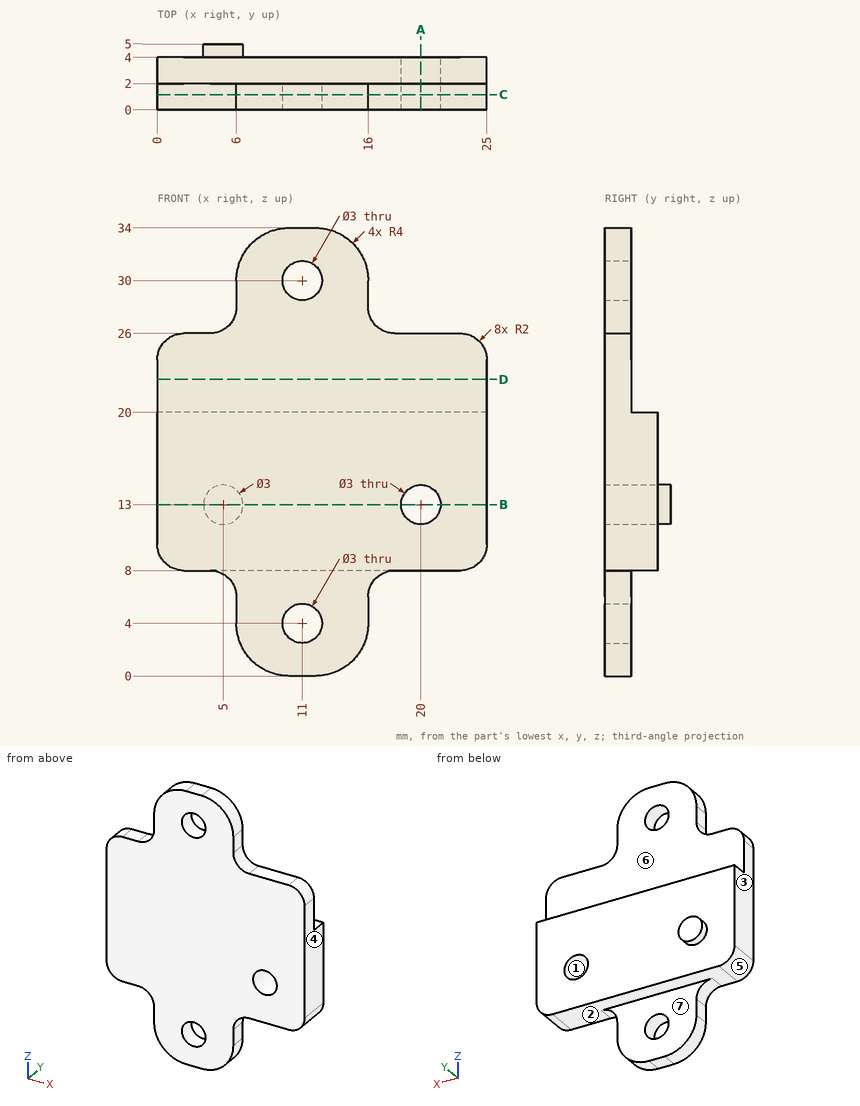
Verification items for this drawing (mm, ordinates from the low corner). A direction names the side the tool comes from. Round coordinates to 2 decimals unless told otherwise and drop trailing zeros. Loops run counter-clockwise (first coordinate to the right, second up) from the corner with the lowest first, then second, coordinate; pieces in that order, holes last. Notation, with made-up numbers: M 2,-18 L 55,-18 A12 ccw 55,-12 Z; hole C -37,30.25 d3. An arc over 180 degrees is marked long. Answer as a JSON object with one key per item and string values.
1. Mould release check, pull along X, two halves, no side actions. Record for the marked faces 1, 2, 3 and 4: pulls with the +X half, pulls with the -X half, needs draft (parallel to the pull), parting line crosses it, or undercut.
Reply:
{"face 1": "undercut", "face 2": "needs draft", "face 3": "pulls with the -X half", "face 4": "pulls with the +X half"}
2. Section check B-B (z = 13). Record the boundary of the cut face in (x, y), plus the area to 3 significant figures.
Reply:
{"outline": "M 0,0 L 18.5,0 L 18.5,4 L 6.5,4 L 6.5,5 L 3.5,5 L 3.5,4 L 0,4 Z; M 21.5,0 L 25,0 L 25,4 L 21.5,4 Z", "area": "91.0 mm²"}
3. Section check C-C (y = 1.15). Record the boundary of the cut face in (x, z), plus the area to 3 significant figures.
Reply:
{"outline": "M 0,10 A2 ccw 2,8 L 4,8 A2 cw 6,6 L 6,4 A4 ccw 10,0 L 12,0 A4 ccw 16,4 L 16,6 A2 cw 18,8 L 23,8 A2 ccw 25,10 L 25,24 A2 ccw 23,26 L 18,26 A2 cw 16,28 L 16,30 A4 ccw 12,34 L 10,34 A4 ccw 6,30 L 6,28 A2 cw 4,26 L 2,26 A2 ccw 0,24 Z; hole C 11,4 d3; hole C 11,30 d3; hole C 20,13 d3", "area": "575 mm²"}
4. Section check A-A (x = 20). Record the boundary of the cut face in (y, z).
Reply:
{"outline": "M 0,8 L 4,8 L 4,11.5 L 0,11.5 Z; M 0,14.5 L 4,14.5 L 4,20 L 2,20 L 2,26 L 0,26 Z"}
5. Scan lines: line 1 (Z direction, x = 11, y = 0.8); line 2 (X direction, y = 0.85, z = 30); line 3 (X direction, y = 1.65, z = 13). Record each from-to range of solid material in increasing order.
Reply:
{"line 1": "z = 0 to 2.5, 5.5 to 28.5, 31.5 to 34", "line 2": "x = 6 to 9.5, 12.5 to 16", "line 3": "x = 0 to 18.5, 21.5 to 25"}
6. Gauge pin test, flat ends, axial feed: P1, Ø1, axis at y = 1, z = 5.5, coming from the -X side; P2, Ø1.5, axis at y = 2, z = 6.5, coming from the +X side; P3, Ø2.5, axis at x = 11, z = 4, coming from the +Y side; P4, Ø3, axis at y = 4.5, z = 7, coming from the +X side. Record the tip position at first contact, or that the pin passes through.
Reply:
{"P1": "stops at x = 6", "P2": "stops at x = 16.44", "P3": "passes through", "P4": "stops at x = 24.22"}
7. Access from +Z, -Z, +X, -X, +Y, -Y to the whole of each face (thin tool, end or side, straight path). Record for the marked faces 5, 6 and 7.
Reply:
{"face 5": "-Z, -X, +Y, -Y", "face 6": "+Z, +X, -X, +Y", "face 7": "-Z, +X, -X, +Y"}
8. Section check D-D (z = 22.5). Record the boundary of the cut face in (x, y).
Reply:
{"outline": "M 0,0 L 25,0 L 25,2 L 0,2 Z"}
